Verification items for the finished model (mm, model axes). A direction names the side the tool comes from. Round coordinates to 2 decimals unless told otherwise and drop trailing zeros. Write each loop counter-clockwise with the first axis right and the second up, starting at its lowest first coordinate (ties: lowest second). Pieces come first, ordered by that corner, then holes.
from build123d import *

# Parameters (mm, degrees)
F0_R     = 10
F1_DEPTH = 1
F2_R     = 10
F2_R_2   = 8.4
F3_DEPTH = 29
F6_DEPTH = 1.6
F7_R     = 1
F8_DEPTH = 1.6
F9_R     = 4
F10_R    = 1


with BuildPart() as f1:
    # F0 (on Top) → F1 (new body)
    with BuildSketch(Plane.XY):
        Circle(F0_R)
    extrude(amount=F1_DEPTH)

    # F2 (on face) → F3 (join)
    with BuildSketch(Plane.XY.offset(1)):
        Circle(F2_R)
        Circle(F2_R_2, mode=Mode.SUBTRACT)
    extrude(amount=F3_DEPTH)

    # F5 (on offset) → F6 (join)
    with BuildSketch(Plane.YZ.offset(10)):
        Polygon((0, 20), (0, 0), (10, 0), (21.547005, 20), align=None)
    extrude(amount=-F6_DEPTH)

    # F7 (on face) → F8 (cut, through all)
    with BuildSketch(Plane.YZ.offset(10)):
        with Locations((13, 16.4)):
            Circle(F7_R)
    extrude(amount=-F8_DEPTH, mode=Mode.SUBTRACT)

    # F9
    f9_edges = [f1.edges().sort_by_distance(p)[0] for p in [
        (9.2, 21.547005, 20),
        (9.2, 10, 0),
    ]]
    fillet(f9_edges, radius=F9_R)

    # F10
    f10_edges = [f1.edges().sort_by_distance(p)[0] for p in [
        (8.4, 5.425864, 10),
    ]]
    fillet(f10_edges, radius=F10_R)


solid = f1.part
Q1. Release check for a two-part mould opening along Y. For faces 4 (the flat face through (9, 9, 20)), 5 (the flat face through (0, 0, 1)), 6 (the cylindrical face through (8.012, 2.523, 15.297)), 7 (the flat face through (9.211, 14.57, 7.916)) record: released by +Y, released by -Y, zero draft, split by the parting line, or undercut.
Recorded:
face 4: zero draft
face 5: undercut
face 6: undercut
face 7: released by +Y
Q2. Material ranges on line 1 along Y through (x, z) = (0, 8); line 2 along Z through (x, y) = (-5.75, -4.5); line 3 along X through (y, z) = (11.25, 9), recorded low to high.
Recorded:
line 1: y = -10 to -8.4, 8.4 to 10
line 2: z = 0 to 1
line 3: x = 8.4 to 10
Q3. Depth check by flat-ended pin: P1, Ø10, axis at x = -6.5, z = 8, coming from the +Y side; P2, Ø8.5, axis at y = 14.5, z = 12, coming from the -X side; P3, Ø3.5, axis at x = 8.5, y = 9.5, coming from the +Z side. Enter the tip coordinate at first touch or a pass-through.
Recorded:
P1: stops at y = 9.89
P2: stops at x = 8.4
P3: stops at z = 20
Q4. Tool access check on faces 1 (the cylindrical face through (9.135, 9.665, 0.521)), 2 (the flat face through (8.4, 12, 12)), 3 (the cylindrical face through (9.19, 18.11, 17.95)). Record the directions out of +Z, -Z, +X, -X, +Y, -Y that give a thin tool (end or side, any length) a straight path to the whole face; none if there is none.
Recorded:
face 1: -Z, +X, +Y
face 2: +Z, -Z, +Y
face 3: +X, -X, +Y
Q5. Sectioned sample at A-A (z = 16.4). Enter the section's corners in (x, y).
Recorded:
outline: (6.73, 7.4) arc R10 ccw (long way) to (10, 0) - (10, 12) - (8.4, 12) - (8.4, 8.14) arc R1 cw to start; (8.4, 14) - (10, 14) - (10, 18.6) - (8.4, 18.6) - close; hole circle Ø16.8 at (0, 0)
Q6. Sectioned sample at B-B (x = 0). Enter the section's corners in (y, z), plus the area to 3 significant figures.
Recorded:
outline: (-10, 0) - (10, 0) - (10, 30) - (8.4, 30) - (8.4, 1) - (-8.4, 1) - (-8.4, 30) - (-10, 30) - close
area: 113 mm2
Q7. Sectioned sample at C-C (y = 2). Enter the section's corners in (x, z), plus the area to 3 significant figures.
Recorded:
outline: (-9.8, 0) - (10, 0) - (10, 20) - (9.8, 20) - (9.8, 30) - (8.16, 30) - (8.16, 1) - (-8.16, 1) - (-8.16, 30) - (-9.8, 30) - close
area: 119 mm2
Q8. Sectioned sample at D-D (y = 13). Enter the section's corners in (x, z).
Recorded:
outline: (8.4, 5.2) - (10, 5.2) - (10, 15.4) - (8.4, 15.4) - close; (8.4, 17.4) - (10, 17.4) - (10, 20) - (8.4, 20) - close
